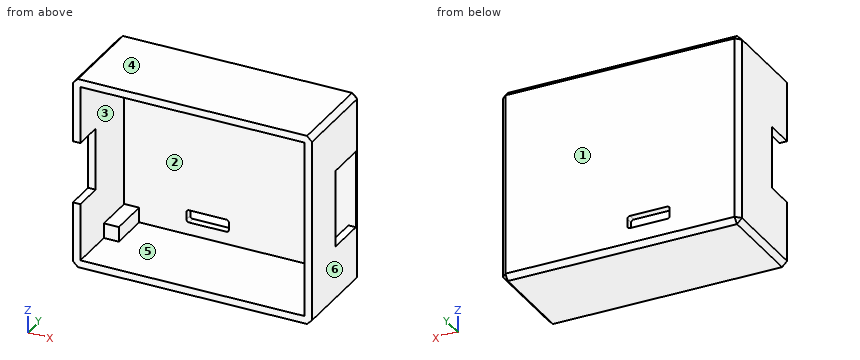
```python
from build123d import *

# Parameters (mm, degrees)
SKETCH2_W           = 24.384
SKETCH2_H           = 19.558
BOSS_EXTRUDE1_DEPTH = 6.477
SKETCH1_W           = 22.86
SKETCH1_H           = 18.034
CUT_EXTRUDE1_DEPTH  = 5.715
SKETCH3_W           = 24.384
SKETCH3_H           = 19.558
SKETCH3_W_2         = 22.86
SKETCH3_H_2         = 18.034
BOSS_EXTRUDE2_DEPTH = 3.048
CUT_EXTRUDE2_REACH  = 33.461
SKETCH4_W           = 6.35
SKETCH4_H           = 6.096
CUT_EXTRUDE3_REACH  = 33.461
SKETCH5_W           = 7.874
SKETCH5_H           = 4.064
CHAMFER1_SIZE       = 0.508
CUT_EXTRUDE4_REACH  = 33.655
SKETCH7_W           = 1.524
SKETCH7_H           = 1.524
BOSS_EXTRUDE3_DEPTH = 4.064


with BuildPart() as part:
    # Sketch2 → Boss-Extrude1 (new body)
    with BuildSketch(Plane(origin=(0, 0, 0), x_dir=(1, 0, 0), z_dir=(0, 1, 0))):
        with Locations((11.43, 9.017)):
            Rectangle(SKETCH2_W, SKETCH2_H)
    extrude(amount=BOSS_EXTRUDE1_DEPTH)

    # Sketch1 → Cut-Extrude1 (cut)
    with BuildSketch(Plane(origin=(0, 0, 0), x_dir=(1, 0, 0), z_dir=(0, 1, 0))):
        with Locations((11.43, 9.017)):
            Rectangle(SKETCH1_W, SKETCH1_H)
    extrude(amount=CUT_EXTRUDE1_DEPTH, mode=Mode.SUBTRACT)

    # Sketch3 → Boss-Extrude2 (add)
    with BuildSketch(Plane.XZ):
        with Locations((11.43, -9.017)):
            Rectangle(SKETCH3_W, SKETCH3_H)
        with Locations((11.43, -9.017)):
            Rectangle(SKETCH3_W_2, SKETCH3_H_2, mode=Mode.SUBTRACT)
    extrude(amount=BOSS_EXTRUDE2_DEPTH)

    # Sketch4 → Cut-Extrude2 (cut, up to next)
    with BuildSketch(Plane.ZY.offset(0.762), mode=Mode.PRIVATE) as cut_extrude2_sk1:
        with Locations((-9.017, -3.048)):
            Rectangle(SKETCH4_W, SKETCH4_H)
    cut_extrude2_tool1 = extrude(cut_extrude2_sk1.sketch, amount=-CUT_EXTRUDE2_REACH, mode=Mode.PRIVATE) & part.part
    add(cut_extrude2_tool1.solids().sort_by_distance((-0.762, -3.048, -9.017))[0], mode=Mode.SUBTRACT)

    # Sketch5 → Cut-Extrude3 (cut, up to next)
    with BuildSketch(Plane(origin=(23.622, 0, 0), x_dir=(0, 0, -1), z_dir=(1, 0, 0)), mode=Mode.PRIVATE) as cut_extrude3_sk1:
        with Locations((9.017, 3.683)):
            Rectangle(SKETCH5_W, SKETCH5_H)
    cut_extrude3_tool1 = extrude(cut_extrude3_sk1.sketch, amount=-CUT_EXTRUDE3_REACH, mode=Mode.PRIVATE) & part.part
    add(cut_extrude3_tool1.solids().sort_by_distance((23.622, 3.683, -9.017))[0], mode=Mode.SUBTRACT)

    # Chamfer1
    chamfer1_edges = [part.edges().sort_by_distance(p)[0] for p in [
        (23.622, 6.477, -9.017),
        (11.43, 6.477, -18.796),
        (-0.762, 6.477, -9.017),
        (11.43, 6.477, 0.762),
        (-0.762, 1.7145, -18.796),
        (23.622, 1.7145, -18.796),
        (23.622, 1.7145, 0.762),
        (-0.762, 1.7145, 0.762),
    ]]
    chamfer(chamfer1_edges, length=CHAMFER1_SIZE)

    # Sketch6 → Cut-Extrude4 (cut, up to next)
    with BuildSketch(Plane(origin=(0, 6.477, 0), x_dir=(1, 0, 0), z_dir=(0, 1, 0)), mode=Mode.PRIVATE) as cut_extrude4_sk1:
        with BuildLine():
            Line((6.604, 16.764), (10.414, 16.764))
            ThreePointArc((10.414, 16.764), (10.593605122, 16.689605122), (10.668, 16.51))
            Line((10.668, 16.51), (10.668, 15.748))
            ThreePointArc((10.668, 15.748), (10.593605122, 15.568394878), (10.414, 15.494))
            Line((10.414, 15.494), (6.604, 15.494))
            ThreePointArc((6.604, 15.494), (6.424394878, 15.568394878), (6.35, 15.748))
            Line((6.35, 15.748), (6.35, 16.51))
            ThreePointArc((6.35, 16.51), (6.424394878, 16.689605122), (6.604, 16.764))
        make_face()
    cut_extrude4_tool1 = extrude(cut_extrude4_sk1.sketch, amount=-CUT_EXTRUDE4_REACH, mode=Mode.PRIVATE) & part.part
    add(cut_extrude4_tool1.solids().sort_by_distance((8.509, 6.477, -16.129))[0], mode=Mode.SUBTRACT)

    # Sketch7 → Boss-Extrude3 (add)
    with BuildSketch(Plane.XZ.offset(-5.715)):
        with Locations((0.762, -17.272)):
            Rectangle(SKETCH7_W, SKETCH7_H)
        with Locations((0.762, -0.762)):
            Rectangle(SKETCH7_W, SKETCH7_H)
    extrude(amount=BOSS_EXTRUDE3_DEPTH)


solid = part.part
```
Geometry check sheet. Reference: the model listing, model coordinates, mm. Face numbers are marked on the shaded views. A direction names the side the tool comes from. Give positions to 0.01 mm unless a question says otherwise; leave off trailing zeros. Write each loop counter-clockwise with the first axis right and the second up, starting at its lowest first coordinate (ties: lowest second). Pieces come first, ordered by that corner, then holes. Notation, with made-up numbers: (63.5, 28.25) -> (88.5, 28.25) arc R20 ccw to (88.5, 58.25) -> close; hole circle Ø6 at (19.5, -21.5). An arc over 180 degrees is marked (long way). One line per question, with ' | ' between items.
Item 1: Depth check by flat-ended pin: pin 1 (0.8 mm diameter, centred on x = 1, z = -1, fed in from -Y); pin 2 (1.5 mm diameter, centred on y = -2, z = -9.5, fed in from -X); pin 3 (9 mm diameter, centred on x = 11.5, z = -11, fed in from -Y) (3 decimals). Enter the tip coordinate at first touch or a pass-through.
Determined:
pin 1: y = 1.65 | pin 2: x = 22.86 | pin 3: y = 5.715
Item 2: Sectioned sample at B-B, the plane x = 7.25. Record the boundary of the cut face in (y, z) (3 decimals), plus the area to 3 significant figures.
Determined:
outline: (-3.048, -18.796) -> (5.969, -18.796) -> (6.477, -18.288) -> (6.477, -16.764) -> (5.715, -16.764) -> (5.715, -18.034) -> (-3.048, -18.034) -> close; (-3.048, 0) -> (5.715, 0) -> (5.715, -15.494) -> (6.477, -15.494) -> (6.477, 0.254) -> (5.969, 0.762) -> (-3.048, 0.762) -> close | area: 27.0 mm^2
Item 3: Sectioned sample at C-C, the plane y = 1. Record the boundary of the cut face in (x, z).
Determined:
outline: (-0.76, -18.29) -> (-0.25, -18.8) -> (23.11, -18.8) -> (23.62, -18.29) -> (23.62, 0.25) -> (23.11, 0.76) -> (-0.25, 0.76) -> (-0.76, 0.25) -> close; hole (0, -18.03) -> (22.86, -18.03) -> (22.86, 0) -> (0, 0) -> close
Item 4: Sectioned sample at A-A, the plane z = -10. Record the boundary of the cut face in (x, y) (3 decimals).
Determined:
outline: (-0.762, 0) -> (0, 0) -> (0, 5.715) -> (23.622, 5.715) -> (23.622, 5.969) -> (23.114, 6.477) -> (-0.254, 6.477) -> (-0.762, 5.969) -> close; (22.86, -3.048) -> (23.622, -3.048) -> (23.622, 1.651) -> (22.86, 1.651) -> close
Item 5: Sectioned sample at D-D, the plane x = 11. Record the boundary of the cut face in (y, z) (3 decimals), plus the area to 3 significant figures.
Determined:
outline: (-3.048, -18.796) -> (5.969, -18.796) -> (6.477, -18.288) -> (6.477, 0.254) -> (5.969, 0.762) -> (-3.048, 0.762) -> (-3.048, 0) -> (5.715, 0) -> (5.715, -18.034) -> (-3.048, -18.034) -> close | area: 28.0 mm^2
Item 6: Access from +Z, -Z, +X, -X, +Y, -Y to the whole of each face (thin tool, end or side, straight path). Record for the marked faces 5 and 6.
Determined:
face 5: -Y | face 6: +Z, -Z, +X, +Y, -Y
Item 7: Scan lines: line 1 along Z through (x, y) = (13.5, -2); line 2 along X through (y, z) = (0.25, -1.75); line 3 along X through (y, z) = (2, -17.25). Record each from-to range of solid material in increasing order.
Determined:
line 1: -18.8 to -18.03, 0 to 0.76 | line 2: -0.76 to 0, 22.86 to 23.62 | line 3: -0.76 to 1.52, 22.86 to 23.62
Item 8: Draft check along Z on the marked faces 1, 2, 3 and 4. Enter one of: released by +Z, released by -Z, zero draft, split by the parting line, or undercut.
Determined:
face 1: zero draft | face 2: undercut | face 3: undercut | face 4: released by +Z
